Design review of the part shown in the three views and the two pictorial views. Dimensions are in mm from the part's minimum x, y and z. A direction names the side the tool comes from. Give positions to 0.01 mm unless a question says otherwise; leave off trailing zeros. Order: outer loops, then holes, each group sorted by start corner. A loop starts at its lowest first (then second) coordinate and runs counter-clockwise, first axis right, second up.
Item 1: For probe 1 along Z at (x, y) = (80, 54.25); probe 2 along Y at (x, z) = (25, 9); probe 3 along X at (y, z) = (28.5, 27), list the stretches that pass through material, from the lowest coordinate up.
Item 2: Consider section D-D (y = 32). Give the boundary of the cut face in (x, z).
Item 3: Consider section B-B (x = 54.5). Give the boundary of the cut face in (y, z), plus the area to 3 significant figures.
Item 4: For P1, Ø4.5, axis at x = 63, z = 19, coming from the -Y side; P2, Ø2, axis at x = 80, z = 43, coming from the -Y side; P3, Ø1, axis at x = 24.5, y = 6.5, coming from the +Z side; P4, Ø6, axis at x = 80, z = 19, coming from the +Y side, all flat-tipped, find the tip position at first contact; note any pin that passes through.
Item 5: The part is to be moulded in two halves that separate along X. For the marked faces 3, 4 and 5, say which applies: released by +X, released by -X, zero draft, split by the parting line, or undercut.
Item 6: Consider section C-C (y = 45). Give the boundary of the cut face in (x, z), plus the area to 3 significant figures.
Item 7: Machinability: for the marked faces 1 and 2, which of the approach directions +Z, -Z, +X, -X, +Y, -Y give a long, thin tool a straight path to every point of the face, cutting with its end or side? Answer none if there is none.
Item 8: Consider section A-A (z = 31). Give the boundary of the cut face in (x, y).
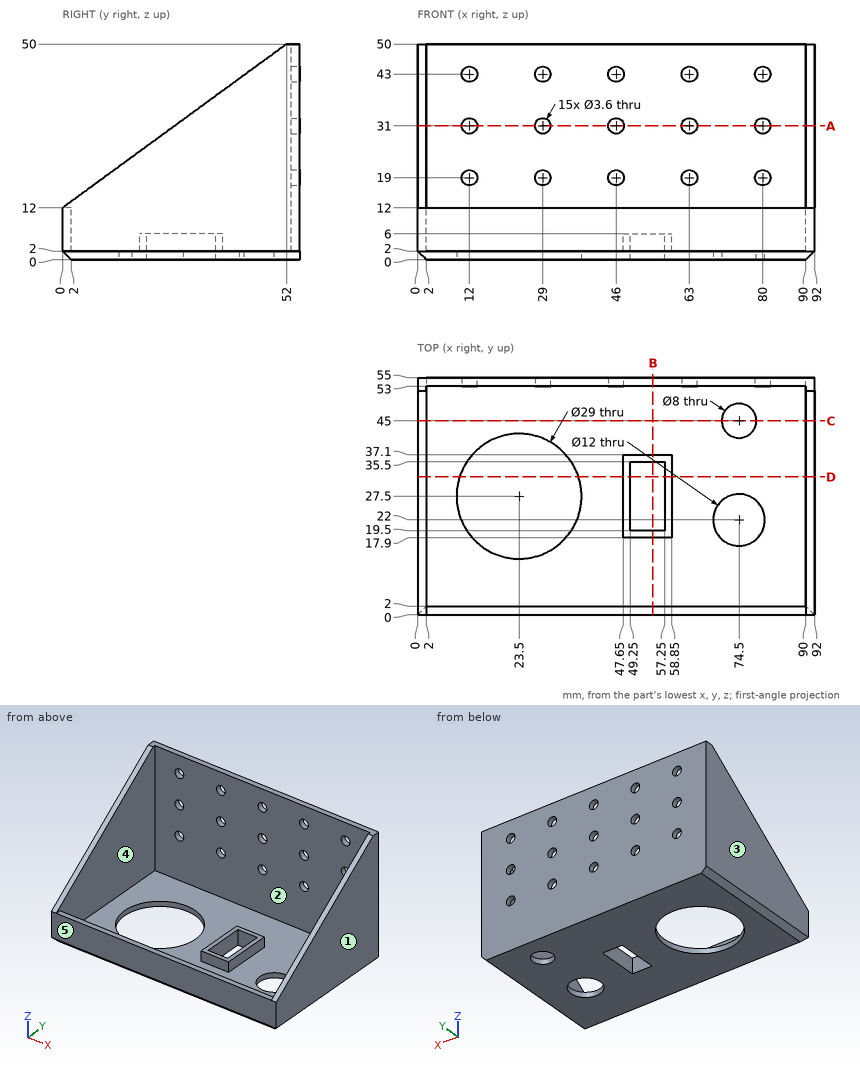
Resolved:
1. probe 1: z = 0 to 17.2, 20.8 to 29.2, 32.8 to 41.2, 44.8 to 50
1. probe 2: y = 0 to 2, 53 to 55
1. probe 3: x = 0 to 2, 90 to 92
2. outline: (0, 2) - (2, 0) - (9.72, 0) - (9.72, 2) - (2, 2) - (2, 35.38) - (0, 35.38) - close; (37.28, 0) - (49.25, 0) - (49.25, 6) - (47.65, 6) - (47.65, 2) - (37.28, 2) - close; (57.25, 0) - (90, 0) - (92, 2) - (92, 35.38) - (90, 35.38) - (90, 2) - (58.85, 2) - (58.85, 6) - (57.25, 6) - close
3. outline: (0, 2) - (2, 0) - (19.5, 0) - (19.5, 6) - (17.9, 6) - (17.9, 2) - (2, 2) - (2, 12) - (0, 12) - close; (35.5, 0) - (55, 0) - (55, 50) - (53, 50) - (53, 2) - (37.1, 2) - (37.1, 6) - (35.5, 6) - close
3. area: 205 mm2
4. P1: stops at y = 53
4. P2: passes through
4. P3: stops at z = 2
4. P4: stops at y = 55
5. face 3: released by -X
5. face 4: undercut
5. face 5: zero draft
6. outline: (0, 2) - (2, 0) - (70.5, 0) - (70.5, 2) - (2, 2) - (2, 44.88) - (0, 44.88) - close; (78.5, 0) - (90, 0) - (92, 2) - (92, 44.88) - (90, 44.88) - (90, 2) - (78.5, 2) - close
6. area: 336 mm2
7. face 1: +Z, -Z, +X, +Y, -Y
7. face 2: +Z
8. outline: (0, 26) - (2, 26) - (2, 53) - (10.2, 53) - (10.2, 55) - (0, 55) - close; (13.8, 53) - (27.2, 53) - (27.2, 55) - (13.8, 55) - close; (30.8, 53) - (44.2, 53) - (44.2, 55) - (30.8, 55) - close; (47.8, 53) - (61.2, 53) - (61.2, 55) - (47.8, 55) - close; (64.8, 53) - (78.2, 53) - (78.2, 55) - (64.8, 55) - close; (81.8, 53) - (90, 53) - (90, 26) - (92, 26) - (92, 55) - (81.8, 55) - close
